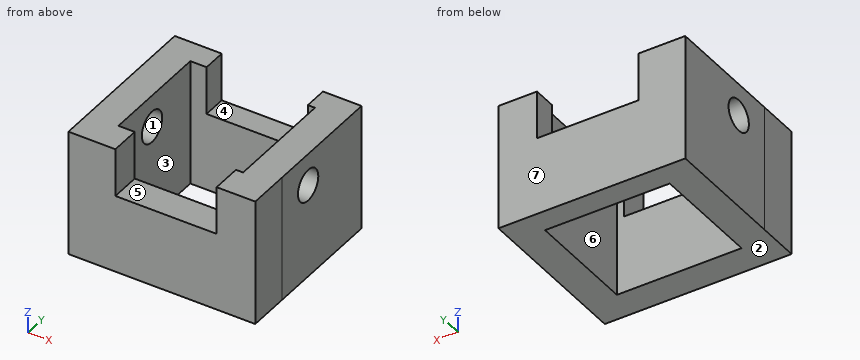
from build123d import *

# Parameters (mm, degrees)
F0_W      = 113.838189
F0_H      = 75.045459
F0_W_2    = 75.969089
F0_H_2    = 47.567274
F1_DEPTH  = 76.962
F1_FACE_W = 113.838188
F1_FACE_H = 76.962
F2_DEPTH  = 25.4
F3_W      = 61.692573
F3_H      = 29.383676
F4_DEPTH  = 132.842
F5_W      = 75.969089
F5_H      = 67.656364
F6_DEPTH  = 129.032
F7_R      = 9.597279
F8_DEPTH  = 241.808


with BuildPart() as f1:
    # F0 (on Top) → F1 (new body)
    with BuildSketch(Plane.XY):
        with Locations((10.044548, 4.618182)):
            Rectangle(F0_W, F0_H)
        with Locations((9.813634, 4.04091)):
            Rectangle(F0_W_2, F0_H_2, mode=Mode.SUBTRACT)
    extrude(amount=F1_DEPTH)

    # F1_face (on face) → F2 (join)
    with BuildSketch(Plane(origin=(10.044549, -32.904547, 38.481), x_dir=(1, 0, 0), z_dir=(0, -1, 0))):
        Rectangle(F1_FACE_W, F1_FACE_H)
    extrude(amount=F2_DEPTH)

    # F3 (on face) → F4 (cut)
    with BuildSketch(Plane.XZ.offset(58.304547)):
        with Locations((12.595225, 62.270162)):
            Rectangle(F3_W, F3_H)
    extrude(amount=-F4_DEPTH, mode=Mode.SUBTRACT)

    # F5 (on Top) → F6 (cut)
    with BuildSketch(Plane.XY):
        with Locations((9.813634, -6.234547)):
            Rectangle(F5_W, F5_H)
    extrude(amount=F6_DEPTH, mode=Mode.SUBTRACT)

    # F7 (on face) → F8 (cut)
    with BuildSketch(Plane.YZ.offset(66.963643)):
        with Locations((-8.354291, 57.352625)):
            Circle(F7_R)
    extrude(amount=-F8_DEPTH, mode=Mode.SUBTRACT)


solid = f1.part
Read the model definition and answer for the solid it produces. Units are mm, in the model's axes. Face numbers are marked on the shaded views. A direction names the side the tool comes from. Round coordinates to 2 decimals unless told otherwise and drop trailing zeros. Write each loop counter-clockwise with the first axis right and the second up, starting at its lowest first coordinate (ties: lowest second). Pieces come first, ordered by that corner, then holes. Notation, with made-up numbers: M -11.5,82.5 L 39.5,82.5 A13 ccw 39.5,101.5 Z; hole C 73.25,83 d11. An arc over 180 degrees is marked long. Use a Markdown table: item, result.
1) Straight lines are drawn through the part: line 1 along X through (y, z) = (4.5, 38); line 2 along X through (y, z) = (-53, 73); line 3 along Y through (x, z) = (-14.5, 34.5). For each, find the intervals that lie inside material, in ascending order. Write a range as [from, to].
Answers follow:
| item | result |
|---|---|
| line 1 | x = [-46.87, -28.17], [47.8, 66.96] |
| line 2 | x = [-46.87, -18.25], [43.44, 66.96] |
| line 3 | y = [-58.3, -40.06], [27.82, 42.14] |
2) The part is cut by section B-B (y = 16). Write down the section's boundary in (x, z).
Answers follow:
| item | result |
|---|---|
| outline | M -46.87,0 L -28.17,0 L -28.17,76.96 L -46.87,76.96 Z; M 47.8,0 L 66.96,0 L 66.96,76.96 L 47.8,76.96 Z |
3) A flat-ended cylindrical pin translates along its axis: pin 1 (1.5 mm diameter, centred on x = 26, y = -44.5, fed in from +Z). Find the tip coordinate at first contact, or state that the pin passes through.
Answers follow:
| item | result |
|---|---|
| pin 1 | stops at z = 47.58 |
4) The part is cut by section C-C (x = 38.5). Write down the section's boundary in (y, z).
Answers follow:
| item | result |
|---|---|
| outline | M -58.3,0 L -40.06,0 L -40.06,47.58 L -58.3,47.58 Z; M 27.82,0 L 42.14,0 L 42.14,47.58 L 27.82,47.58 Z |
5) For a pull along Z with two mould halves and no side action, classify the marked faces 1, 2, 3 and 4 as pulls with the +Z half, pulls with the -Z half, needs draft (parallel to the pull), parting line crosses it, or undercut.
Answers follow:
| item | result |
|---|---|
| face 1 | undercut |
| face 2 | pulls with the -Z half |
| face 3 | needs draft |
| face 4 | pulls with the +Z half |
6) A tool of negligible diameter and unlimited length cuts with its end or side. For the marked faces 5, 6 and 7, from which of +Z, -Z, +X, -X, +Y, -Y can it reach the whole face along a straight path? Write none if from no direction.
Answers follow:
| item | result |
|---|---|
| face 5 | +Z, +Y, -Y |
| face 6 | +Z, -Z |
| face 7 | +Z, -Z, +X, -X, +Y |
